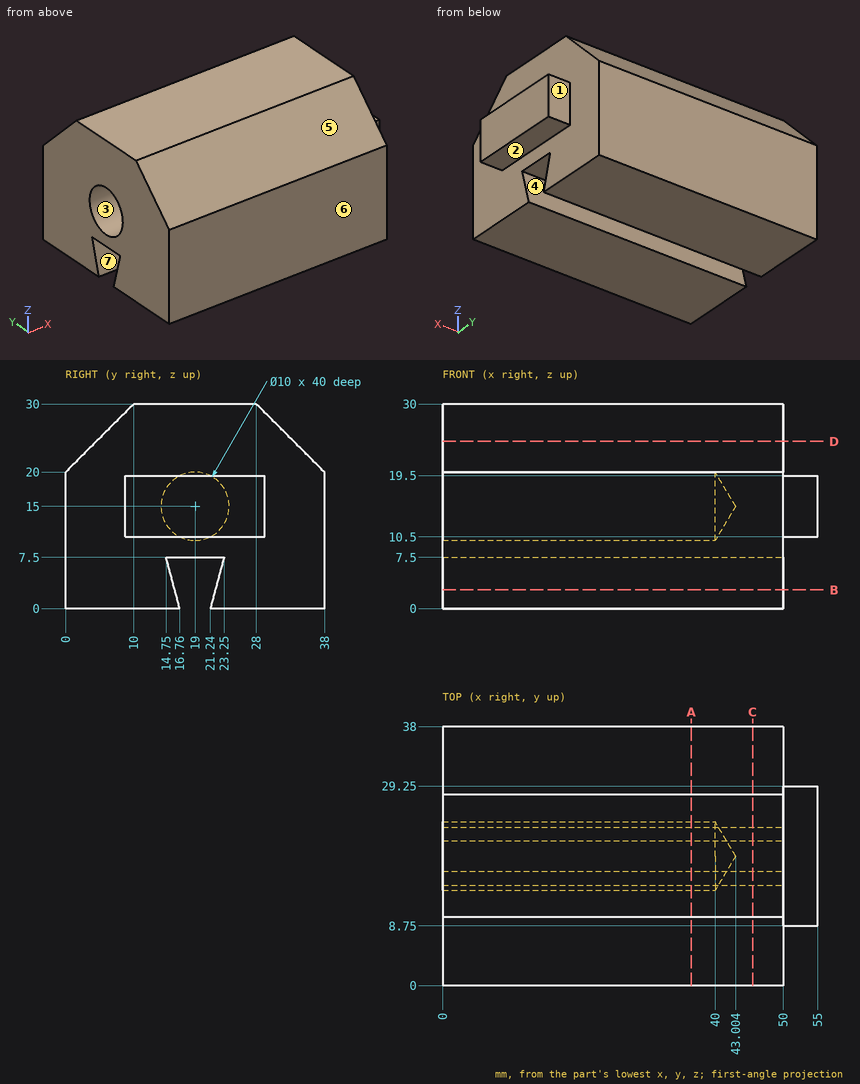
Check sheet for the drawn part. Datum: minimum x, y, z corner. Units: mm. A direction names the side the tool comes from. Give positions to 0.01 mm unless a question says otherwise; leave off trailing zeros. Order: outer loops, then holes, each group sorted by start corner. A loop starts at its lowest first (then second) coordinate and runs counter-clockwise, first axis right, second up. Notation, with made-up numbers: (60.25, 56.25) -> (102.25, 56.25) arc R15 ccw to (102.25, 70.25) -> close; hole circle Ø9 at (-29.75, 56). An arc over 180 degrees is marked (long way). Use a Markdown table: item, result.
1) Material ranges on probe 1 along Y at (x, z) = (21.5, 15); probe 2 along Z at (x, y) = (12.5, 19); probe 3 along X at (y, z) = (30.5, 21), recorded low to high.
Results:
| item | result |
|---|---|
| probe 1 | 0 to 14, 24 to 38 |
| probe 2 | 7.5 to 10, 20 to 30 |
| probe 3 | 0 to 50 |
2) Depth check by flat-ended pin: pin 1 Ø1.5 at (x, z) = (51.5, 13) entering from +Y; pin 2 Ø2.5 at (x, y) = (53, 16.5) entering from -Z; pin 3 Ø10 at (y, z) = (33, 4.5) entering from +X. Enter the tip coordinate at first touch or a pass-through.
Results:
| item | result |
|---|---|
| pin 1 | y = 29.25 |
| pin 2 | z = 10.5 |
| pin 3 | x = 50 |
3) Section check D-D, the plane z = 24.5. Record the boundary of the cut face in (x, y), then the cut area to 3 significant figures.
Results:
| item | result |
|---|---|
| outline | (0, 4.5) -> (50, 4.5) -> (50, 33.5) -> (0, 33.5) -> close |
| area | 1,450 mm² |
4) Mould release check, pull along Z, two halves, no side actions. Record for the marked faces 5, 6 and 7: pulls with the +Z half, pulls with the -Z half, needs draft (parallel to the pull), parting line crosses it, or undercut.
Results:
| item | result |
|---|---|
| face 5 | pulls with the +Z half |
| face 6 | needs draft |
| face 7 | undercut |
5) Section check B-B, the plane z = 2.75. Record the boundary of the cut face in (x, y).
Results:
| item | result |
|---|---|
| outline | (0, 0) -> (50, 0) -> (50, 16.02) -> (0, 16.02) -> close; (0, 21.98) -> (50, 21.98) -> (50, 38) -> (0, 38) -> close |
6) Section check A-A, the plane x = 36.5. Record the boundary of the cut face in (y, z), then the cut area to 3 significant figures.
Results:
| item | result |
|---|---|
| outline | (0, 0) -> (16.76, 0) -> (14.75, 7.5) -> (23.25, 7.5) -> (21.24, 0) -> (38, 0) -> (38, 20) -> (28, 30) -> (10, 30) -> (0, 20) -> close; hole circle Ø10 at (19, 15) |
| area | 913 mm² |
7) Tool access check on the marked faces 1, 2, 3 and 4. Record the directions out of +Z, -Z, +X, -X, +Y, -Y that give a thin tool (end or side, any length) a straight path to the whole face; none if there is none.
Results:
| item | result |
|---|---|
| face 1 | +Z, -Z, +X, +Y |
| face 2 | -Z, +X, +Y, -Y |
| face 3 | -X |
| face 4 | +X, -X |
8) Section check C-C, the plane x = 45.5. Record the boundary of the cut face in (y, z).
Results:
| item | result |
|---|---|
| outline | (0, 0) -> (16.76, 0) -> (14.75, 7.5) -> (23.25, 7.5) -> (21.24, 0) -> (38, 0) -> (38, 20) -> (28, 30) -> (10, 30) -> (0, 20) -> close |
